Design review of the part built by this model. Coordinates are the model's own, in mm. Face numbers are marked on the shaded views. Coordinates: 2 decimals unless noted, no trailing zeros. Loops run counter-clockwise (first coordinate to the right, second up) from the corner with the lowest first, then second, coordinate; pieces in that order, holes last. Notation, with made-up numbers: (10, 83.5) -> (57, 83.5) arc R29 ccw to (57, 106.5) -> close; hole circle Ø6 at (10.25, 60). An arc over 180 degrees is marked (long way). One line per item, written item: value. Start each with the question number.
1. Add section B-B on y = 13. Write out the cut boundary in (x, z), plus the area to 3 significant figures.
2. Draft analysis for pull direction X (two halves, no side actions). For the marked faces 1, 2 and 3, state which applies: pulls with the +X half, pulls with the -X half, needs draft (parallel to the pull), parting line crosses it, or undercut.
3. Insertion check: pin 1 (2 mm diameter, centred on x = -4, y = 38.5, fed in from +Z); pin 2 (10 mm diameter, centred on y = 30.5, z = 1.5, fed in from -X); pin 3 (1.2 mm diameter, centred on x = 7, y = 1, fed in from +Z). Each pin has a flat end and moves straight along its axis. Give the tip position at first contact, or say it passes through.
4. For probe 1 along Y at (x, z) = (0, -2.5); probe 2 along X at (y, z) = (3.5, -38.5); probe 3 along X at (y, z) = (11, -46), list the stretches that pass through material, from the lowest coordinate up.
5. Add section A-A on z = -51. Write out the cut boundary in (x, y).
```python
from build123d import *

# Parameters (mm, degrees)
SKETCH1_R           = 1
BOSS_EXTRUDE1_DEPTH = 40
CUT_EXTRUDE2_DEPTH  = 16
SKETCH5_W           = 10
SKETCH5_H           = 13
CUT_EXTRUDE3_DEPTH  = 12.75
BOSS_EXTRUDE2_START = -4
BOSS_EXTRUDE2_DEPTH = 4


# Read off the part's stored shape, not the designer's step: Boss-Extrude2
with BuildPart() as part:
    # Sketch1 → Boss-Extrude1 (new body)
    with BuildSketch(Plane(origin=(0, 0, 0), x_dir=(1, 0, 0), z_dir=(0, 1, 0))):
        with BuildLine():
            Line((10, 0), (0, 60))
            Line((0, 60), (-9.860132972, 1.666666667))
            ThreePointArc((-9.860132972, 1.666666667), (-0.836262603, -9.964971895), (10, 0))
        make_face()
        with BuildLine():
            Line((-8.959471052, -1), (-2.414213562, -1))
            Line((-2.414213562, -1), (-7.042409518, -5.628195955))
            ThreePointArc((-7.042409518, -5.628195955), (-8.328871165, -3.449931396), (-8.959471052, -1))
        make_face(mode=Mode.SUBTRACT)
        with BuildLine():
            Line((-2.414213562, 1), (-8.959471052, 1))
            ThreePointArc((-8.959471052, 1), (-8.328871165, 3.449931396), (-7.042409518, 5.628195955))
            Line((-7.042409518, 5.628195955), (-2.414213562, 1))
        make_face(mode=Mode.SUBTRACT)
        with BuildLine():
            Line((-5.628195955, -7.042409518), (-1, -2.414213562))
            Line((-1, -2.414213562), (-1, -8.959471052))
            ThreePointArc((-1, -8.959471052), (-3.449931396, -8.328871165), (-5.628195955, -7.042409518))
        make_face(mode=Mode.SUBTRACT)
        with BuildLine():
            Line((-1, 8.959471052), (-1, 2.414213562))
            Line((-1, 2.414213562), (-5.628195955, 7.042409518))
            ThreePointArc((-5.628195955, 7.042409518), (-3.449931396, 8.328871165), (-1, 8.959471052))
        make_face(mode=Mode.SUBTRACT)
        with Locations(Location((0, 0, 0), (0, 0, 270))):
            Circle(SKETCH1_R, mode=Mode.SUBTRACT)
        with BuildLine():
            Line((1, -2.414213562), (5.628195955, -7.042409518))
            ThreePointArc((5.628195955, -7.042409518), (3.449931396, -8.328871165), (1, -8.959471052))
            Line((1, -8.959471052), (1, -2.414213562))
        make_face(mode=Mode.SUBTRACT)
        with BuildLine():
            Line((1, 2.414213562), (1, 8.959471052))
            ThreePointArc((1, 8.959471052), (3.449931396, 8.328871165), (5.628195955, 7.042409518))
            Line((5.628195955, 7.042409518), (1, 2.414213562))
        make_face(mode=Mode.SUBTRACT)
        with BuildLine():
            ThreePointArc((8.959471052, -1), (8.328871165, -3.449931396), (7.042409518, -5.628195955))
            Line((7.042409518, -5.628195955), (2.414213562, -1))
            Line((2.414213562, -1), (8.959471052, -1))
        make_face(mode=Mode.SUBTRACT)
        with BuildLine():
            ThreePointArc((7.042409518, 5.628195955), (8.328871165, 3.449931396), (8.959471052, 1))
            ThreePointArc((8.959471052, 1), (9.005377927, 0.418676383), (9.013606076, -0.164398987))
            Line((9.013606076, -0.164398987), (8.819539578, 1))
            Line((8.819539578, 1), (2.414213562, 1))
            Line((2.414213562, 1), (7.042409518, 5.628195955))
        make_face(mode=Mode.SUBTRACT)
        with BuildLine():
            ThreePointArc((7.982280685, 6.023553358), (-0.139863688, 9.99902186), (-8.147636517, 5.797932319))
            Line((-8.147636517, 5.797932319), (-0.006945449, 53.958910167))
            Line((-0.006945449, 53.958910167), (7.982280685, 6.023553358))
        make_face(mode=Mode.SUBTRACT)
    extrude(amount=BOSS_EXTRUDE1_DEPTH)

    # Sketch4 → Cut-Extrude2 (cut, symmetric)
    with BuildSketch(Plane(origin=(0, 20, 0), x_dir=(-1, 0, 0), z_dir=(0, -1, 0))):
        Polygon((-8.978243143, 0.814414874), (-12.501432649, 0.814414874), (-12.501432649, -9.874000046), (27.256185967, -11.315556265), (27.256185967, 53.958910167), (0.006945449, 53.958910167), (-7.982280685, 6.023553358), align=None)
    extrude(amount=CUT_EXTRUDE2_DEPTH, both=True, mode=Mode.SUBTRACT)

    # Sketch5 → Cut-Extrude3 (cut, symmetric)
    with BuildSketch(Plane(origin=(9.72972973, 0, -1.621621622), x_dir=(-0.1643989873053573, 0, -0.9863939238321439), z_dir=(0.9863939238321439, 0, -0.1643989873053573))):
        with Locations((4.181658841, 13.5)):
            Rectangle(SKETCH5_W, SKETCH5_H)
        with Locations((4.181658841, 26.5)):
            Rectangle(SKETCH5_W, SKETCH5_H)
    extrude(amount=CUT_EXTRUDE3_DEPTH, both=True, mode=Mode.SUBTRACT)

    # Boss-Extrude2 outline → Boss-Extrude2 (add)
    with BuildSketch(Plane.XZ.offset(BOSS_EXTRUDE2_START)):
        with BuildLine():
            ThreePointArc((-5.749720089, -19.984197223), (-4.96405921, -19.931964722), (-4.564704551, -20.610571462))
            ThreePointArc((-4.564704551, -20.610571462), (-3.585635952, -21.631073632), (-2.565133782, -20.652005033))
            ThreePointArc((-2.565133782, -20.652005033), (-1.799757155, -19.917703584), (-1.065455705, -20.683080211))
            ThreePointArc((-1.065455705, -20.683080211), (-0.07602927, -21.703743341), (0.934329679, -20.703796997))
            ThreePointArc((0.934329679, -20.703796997), (1.684329679, -19.953796997), (2.434329679, -20.703796997))
            ThreePointArc((2.434329679, -20.703796997), (3.434329679, -21.703796997), (4.434329679, -20.703796997))
            ThreePointArc((4.434329679, -20.703796997), (4.849537937, -20.032667732), (5.635434984, -20.104627568))
            Line((5.635434984, -20.104627568), (5.680296948, -19.83545578))
            ThreePointArc((5.680296948, -19.83545578), (4.644652016, -19.86192526), (4.188222104, -20.791942891))
            Line((4.188222104, -20.791942891), (4.179154082, -20.79175499))
            ThreePointArc((4.179154082, -20.79175499), (3.41879209, -21.453636035), (2.68650098, -20.760825378))
            Line((2.68650098, -20.760825378), (2.682706725, -20.760746756))
            ThreePointArc((2.682706725, -20.760746756), (1.705046464, -19.704011612), (0.684450485, -20.719340424))
            Line((0.684450485, -20.719340424), (0.684168717, -20.719334586))
            ThreePointArc((0.684168717, -20.719334586), (-0.08120791, -21.453636035), (-0.815509359, -20.688259408))
            ThreePointArc((-0.815509359, -20.688259408), (-1.794577958, -19.667757238), (-2.815080128, -20.646825837))
            ThreePointArc((-2.815080128, -20.646825837), (-3.580456755, -21.381127286), (-4.314758204, -20.615750659))
            ThreePointArc((-4.314758204, -20.615750659), (-4.795852318, -19.740072257), (-5.794737363, -19.717871437))
            Line((-5.794737363, -19.717871437), (-5.749720089, -19.984197223))
        make_face()
    boss_extrude2 = extrude(amount=BOSS_EXTRUDE2_DEPTH)

    # Mirror2: Boss-Extrude2 across plane
    add(boss_extrude2.mirror(Plane(origin=(0, 20, 0), x_dir=(0, 0, 1), z_dir=(0, -1, 0))))


solid = part.part
```
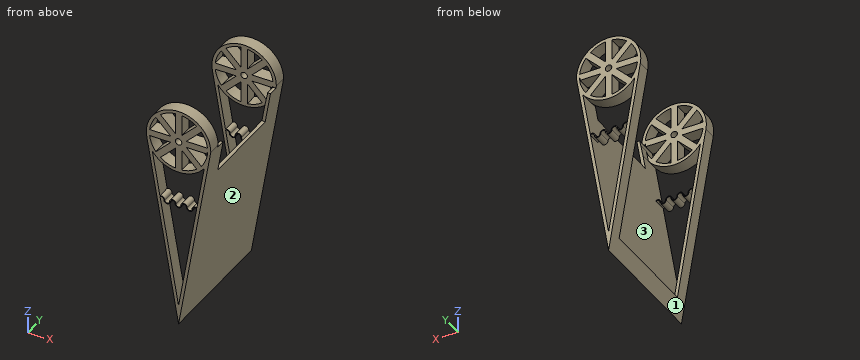
Worked answers:
1. outline: (-1.02, -53.96) -> (0, -60) -> (8.22, -10.68) -> (7.23, -10.51) -> (-0.01, -53.96) -> close
1. area: 50.1 mm²
2. face 1: pulls with the -X half
2. face 2: pulls with the +X half
2. face 3: undercut
3. pin 1: stops at z = 9.54
3. pin 2: stops at x = 8.59
3. pin 3: stops at z = 7.68
4. probe 1: y = 0 to 4, 36 to 40
4. probe 2: x = -3.63 to -2.62, 2.57 to 3.58
4. probe 3: x = 1.32 to 2.33
5. outline: (-1.52, 0) -> (-0.51, 0) -> (-0.51, 4) -> (-1.52, 4) -> close; (-1.52, 36) -> (-0.51, 36) -> (-0.51, 40) -> (-1.52, 40) -> close; (0.49, 0) -> (1.5, 0) -> (1.5, 40) -> (0.49, 40) -> close
